For this review, take the finished solid that the model builds, in its own axes (mm). A direction names the side the tool comes from. Coordinates: 2 decimals unless noted, no trailing zeros. Loops run counter-clockwise (first coordinate to the right, second up) from the corner with the lowest first, then second, coordinate; pieces in that order, holes last. Notation, with made-up numbers: (53.25, -2) -> (72.25, -2) arc R20 ccw to (72.25, 17) -> close; hole circle Ø9 at (55.25, -23). An arc over 180 degrees is marked (long way). Answer in a Markdown table with one row per item.
Autodesk Inventor part; units mm, degrees
ref_plane "YZ Plane" through (0, 0, 0) normal (1, 0, 0) x (0, 1, 0)
ref_plane "XZ Plane" through (0, 0, 0) normal (0, 1, 0) x (-1, 0, 0)
ref_plane "XY Plane" through (0, 0, 0) normal (0, 0, 1) x (1, 0, 0)
sketch "Sketch4" plane through (0, 0, 0) normal (0, 1, 0) x (-1, 0, 0)
  circle A0 centre (0, 0) radius 1.5
  line L0 (-2, 2) -> (2, 2)
  line L1 (2, 2) -> (2, -2)
  line L2 (2, -2) -> (-2, -2)
  line L3 (-2, -2) -> (-2, 2)
  line L4 (-2, 2) -> (2, -2) construction
  line L5 (2, 2) -> (-2, -2) construction
  point P0 (-1.5, 0)
  point P1 (0, -1.5)
  point P2 (0, 1.5)
  point P3 (1.5, 0)
  dimension "Radius" = 3
  dimension "d103" = 4
extrude "Extrusion2" add sketch "Sketch4" along normal mid plane 42 contours A0
extrude "Extrusion10" add sketch "Sketch4" against normal up to surface (21 mm away) contours A0 | L0 L1 L2 L3
chamfer "Chamfer1" distance 0.2 angle 45 9 edges at (1.5, 21, 0) (0, -21, -2) (2, -21, 0) (0, -21, 2) (-2, -21, 0) (2, 0, 0) (0, 0, 2) (-2, 0, 0) (0, 0, -2)
sketch "Sketch14" plane through (2, -0.2, -2) normal (0, 0, -1) x (-1, 0, 0)
  line L0 (0, 0) -> (0, -20.6)
  line L1 (0, -10.3) -> (2, -10.3) construction
  point P0 (2, 0.2)
hole "Hole6" at (0, -10.5, -2) direction (0, 0, 1) diameter 2.459 end through all
properties part number "Ball Track Rest Pin" material "Bronze, Soft Tin"
Item 1: Insertion check: pin 1 (2 mm diameter, centred on x = 1, y = 2.5, fed in from +Z); pin 2 (1.5 mm diameter, centred on y = 8.5, z = -1.5, fed in from +X). Each pin has a flat end and moves straight along its axis. Give the tip position at first contact, or say it passes through.
Worked answers:
| item | result |
|---|---|
| pin 1 | z = 1.5 |
| pin 2 | x = 1.3 |
Item 2: Take a section at C-C, the plane x = 0. State the section outline as (y, z) points, and give its area (3 significant figures).
Worked answers:
| item | result |
|---|---|
| outline | (-21, -1.8) -> (-20.8, -2) -> (-11.73, -2) -> (-11.73, 2) -> (-20.8, 2) -> (-21, 1.8) -> close; (-9.27, -2) -> (-0.2, -2) -> (0, -1.8) -> (0, -1.5) -> (20.8, -1.5) -> (21, -1.3) -> (21, 1.3) -> (20.8, 1.5) -> (0, 1.5) -> (0, 1.8) -> (-0.2, 2) -> (-9.27, 2) -> close |
| area | 137 mm² |
Item 3: Take a section at A-A, the plane y = -10.5. State the section outline as (x, z) points.
Worked answers:
| item | result |
|---|---|
| outline | (-2, -2) -> (-1.23, -2) -> (-1.23, 2) -> (-2, 2) -> close; (1.23, -2) -> (2, -2) -> (2, 2) -> (1.23, 2) -> close |
Item 4: Take a section at D-D, the plane y = 3. State the section outline as (x, z) points, and give its area (3 significant figures).
Worked answers:
| item | result |
|---|---|
| outline | circle Ø3 at (0, 0) |
| area | 7.07 mm² |
Item 5: The part is to be moulded in two halves that separate along Y. For faces 3 (the flat face through (1.4, -10.4, 2)), 4 (the cylindrical face through (-0.369, -9.327, 0.028)), 5 (the flat face through (0, -21, 0)), say which applies: +Y half, -Y half, draft (parallel to the pull), parting line (faces both ways), or undercut.
Worked answers:
| item | result |
|---|---|
| face 3 | draft |
| face 4 | undercut |
| face 5 | -Y half |
Item 6: For faces 1 (the flat face through (0, 21, 0)), 2 (the cylindrical face through (1.5, 10.25, -0.07)), list the 3-axis set-ups (+Z, -Z, +X, -X, +Y, -Y) from which the entire face can be reached by the end or side of a thin tool; tool diameter is ignored.
Worked answers:
| item | result |
|---|---|
| face 1 | +Z, -Z, +X, -X, +Y |
| face 2 | +Y |
Item 7: For L1, parallel to Y at x = 0, z = 0.85; L2, parallel to X at y = -10.5, z = -0.75; L3, parallel to X at y = 9, z = -0.15, list the stretches that pass through material, from the lowest coordinate up.
Worked answers:
| item | result |
|---|---|
| L1 | -21 to -11.73, -9.27 to 21 |
| L2 | -2 to -1.23, 1.23 to 2 |
| L3 | -1.49 to 1.49 |
Item 8: Take a section at B-B, the plane z = 0. State the section outline as (x, y) points.
Worked answers:
| item | result |
|---|---|
| outline | (-2, -20.8) -> (-1.8, -21) -> (1.8, -21) -> (2, -20.8) -> (2, -0.2) -> (1.8, 0) -> (1.5, 0) -> (1.5, 20.8) -> (1.3, 21) -> (-1.3, 21) -> (-1.5, 20.8) -> (-1.5, 0) -> (-1.8, 0) -> (-2, -0.2) -> close; hole circle Ø2.46 at (0, -10.5) |
